from build123d import *

# Parameters (mm, degrees)
F0_W     = 400
F0_H     = 400
F0_R     = 2.5
F0_R_2   = 10.228348
F0_R_3   = 50
F0_R_4   = 10
F1_DEPTH = 25
F2_R     = 5
F3_DEPTH = 100


with BuildPart() as f1:
    # F0 (on Front) → F1 (new body)
    with BuildSketch(Plane.XZ):
        with Locations((-11.235014, 3.358459)):
            Rectangle(F0_W, F0_H)
        with Locations((-182.950743, -168.35727)):
            Circle(F0_R, mode=Mode.SUBTRACT)
        with Locations((-175.879675, -161.286202)):
            Circle(F0_R, mode=Mode.SUBTRACT)
        with Locations((-169.089688, -168.157667)):
            Circle(F0_R, mode=Mode.SUBTRACT)
        with Locations((-161.782501, -161.33088)):
            Circle(F0_R, mode=Mode.SUBTRACT)
        with Locations((-182.950743, -154.215134)):
            Circle(F0_R, mode=Mode.SUBTRACT)
        with Locations((-175.879614, -147.144127)):
            Circle(F0_R, mode=Mode.SUBTRACT)
        with Locations((-168.808607, -154.215134)):
            Circle(F0_R, mode=Mode.SUBTRACT)
        with Locations((-154.809286, -168.498464)):
            Circle(F0_R, mode=Mode.SUBTRACT)
        with Locations((-182.98271, -140.105038)):
            Circle(F0_R, mode=Mode.SUBTRACT)
        with Locations((-78.123887, -63.530414)):
            Circle(F0_R_2, mode=Mode.SUBTRACT)
        with Locations((-78.997388, 71.41491)):
            Circle(F0_R_3, mode=Mode.SUBTRACT)
        with Locations((-183.240077, 147.128803)):
            Circle(F0_R, mode=Mode.SUBTRACT)
        with Locations((-176.072493, 154.102018)):
            Circle(F0_R, mode=Mode.SUBTRACT)
        with Locations((-182.89928, 161.409204)):
            Circle(F0_R, mode=Mode.SUBTRACT)
        with Locations((-168.956747, 161.128124)):
            Circle(F0_R, mode=Mode.SUBTRACT)
        with Locations((-176.027815, 168.199192)):
            Circle(F0_R, mode=Mode.SUBTRACT)
        with Locations((-182.92664, 175.098311)):
            Circle(F0_R, mode=Mode.SUBTRACT)
        with Locations((-161.88574, 168.199131)):
            Circle(F0_R, mode=Mode.SUBTRACT)
        with Locations((-168.956747, 175.270259)):
            Circle(F0_R, mode=Mode.SUBTRACT)
        with Locations((-154.475159, 174.922457)):
            Circle(F0_R, mode=Mode.SUBTRACT)
        with Locations((55.839185, 70.432658)):
            Circle(F0_R_4, mode=Mode.SUBTRACT)
        with Locations((160.530572, 146.804111)):
            Circle(F0_R, mode=Mode.SUBTRACT)
        with Locations((131.988816, 174.482275)):
            Circle(F0_R, mode=Mode.SUBTRACT)
        with Locations((146.356469, 160.914207)):
            Circle(F0_R, mode=Mode.SUBTRACT)
        with Locations((153.427477, 153.8432)):
            Circle(F0_R, mode=Mode.SUBTRACT)
        with Locations((160.498605, 160.914207)):
            Circle(F0_R, mode=Mode.SUBTRACT)
        with Locations((139.279189, 167.637536)):
            Circle(F0_R, mode=Mode.SUBTRACT)
        with Locations((145.93778, 175.098311)):
            Circle(F0_R, mode=Mode.SUBTRACT)
        with Locations((153.427537, 167.985275)):
            Circle(F0_R, mode=Mode.SUBTRACT)
        with Locations((160.480715, 175.074188)):
            Circle(F0_R, mode=Mode.SUBTRACT)
    extrude(amount=F1_DEPTH)

    # F2
    f2_edges = [f1.edges().sort_by_distance(p)[0] for p in [
        (-128.997388, 0, 71.41491),
        (-128.997388, -25, 71.41491),
    ]]
    fillet(f2_edges, radius=F2_R)

    # F0 (on Front) → F3 (join)
    with BuildSketch(Plane.XZ):
        with Locations((55.839185, 70.432658)):
            Circle(F0_R_4)
        with Locations((-78.123887, -63.530414)):
            Circle(F0_R_2)
    extrude(amount=F3_DEPTH)


solid = f1.part
Geometry: final body of the model. Coordinates: model frame, mm. A direction names the side the tool comes from. Give positions to 0.01 mm unless a question says otherwise; leave off trailing zeros. Order: outer loops, then holes, each group sorted by start corner. A loop starts at its lowest first (then second) coordinate and runs counter-clockwise, first axis right, second up. Notation, with made-up numbers: (-26.5, 5.25) -> (31.5, 5.25) arc R22 cw to (31.5, 35.25) -> close; hole circle Ø6 at (20, 55.5). An arc over 180 degrees is marked (long way). Answer as a JSON object with one key per item and string values.
Q1. Material intervals for probe 1 along Z at (x, y) = (153, -11); probe 2 along Z at (x, y) = (-175.5, -13.5); probe 3 along Z at (x, y) = (-111, -17.5), sorted ascending.
Entries:
{"probe 1": "z = -196.64 to 151.38, 156.31 to 165.52, 170.45 to 203.36", "probe 2": "z = -196.64 to -163.76, -158.82 to -149.62, -144.67 to 151.67, 156.54 to 165.76, 170.64 to 203.36", "probe 3": "z = -196.64 to 33, 109.83 to 203.36"}
Q2. Section B-B (z = -42.5). Output: boundary loops of the cut face in (x, y).
Entries:
{"outline": "(-211.24, -25) -> (188.76, -25) -> (188.76, 0) -> (-211.24, 0) -> close"}
Q3. Section C-C (y = -13.5). State how many separate pieces and enclosed holes the cut face has, plus the area to 3 significant figures.
Entries:
{"separate pieces": "1", "enclosed holes": "28", "area": "152,000 mm^2"}
Q4. Access query for faces 1 (the flat face through (-78, -100, -63)), 2 (the cylindrical face through (54.537, -61.975, 80.348)). Directions: +Z, -Z, +X, -X, +Y, -Y. A direction counts if a zero-diameter tool reaches every point of the face in a straight line with its end or side. Return the directions, or none.
Entries:
{"face 1": "+Z, -Z, +X, -X, -Y", "face 2": "-Y"}
Q5. Section D-D (y = -72). Output: boundary loops of the cut face in (x, z), plus the area to 3 significant figures.
Entries:
{"outline": "circle Ø20.46 at (-78.12, -63.53); circle Ø20 at (55.84, 70.43)", "area": "643 mm^2"}
Q6. Draft query along Z for faces 3 (the cylindrical face through (-115.849, -12.395, 105.207)), 4 (the flat face through (-211.235, -12, 1)), 5 (the cylindrical face through (-73.404, -61.975, -72.605)). Return one class per face: released by +Z, released by -Z, zero draft, split by the parting line, or undercut.
Entries:
{"face 3": "undercut", "face 4": "zero draft", "face 5": "split by the parting line"}
Q7. Section A-A (x = 58). Output: boundary loops of the cut face in (y, z).
Entries:
{"outline": "(-100, 60.67) -> (-25, 60.67) -> (-25, -196.64) -> (0, -196.64) -> (0, 203.36) -> (-25, 203.36) -> (-25, 80.2) -> (-100, 80.2) -> close"}
Q8. First-contact query: pin 1 (8 mm diameter, centred on x = -168.81, z = -154.22, fed in from +Y); pin 2 (6.5 mm diameter, centred on x = -169.09, z = -168.16, fed in from -Y); pin 3 (4 mm diameter, centred on x = -77, y = -43, fed in from +Z). Flat tips, straight axial feed; report the tip coordinate or a pass-through.
Entries:
{"pin 1": "stops at y = 0", "pin 2": "stops at y = -25", "pin 3": "stops at z = -53.3"}
